Could you check a few things on this drawing? It's one solid part, dimensions in mm from its lowest x, y, z. Round coordinates to 2 decimals unless told otherwise and drop trailing zeros. Loops run counter-clockwise (first coordinate to the right, second up) from the corner with the lowest first, then second, coordinate; pieces in that order, holes last. Notation, with made-up numbers: (-39.5, 68.25) -> (-34.5, 68.25) arc R24 cw to (-34.5, 102.25) -> close; hole circle Ø5 at (15, 62). An arc over 180 degrees is marked (long way). Write each question's results on one line, items separated by ' | '.
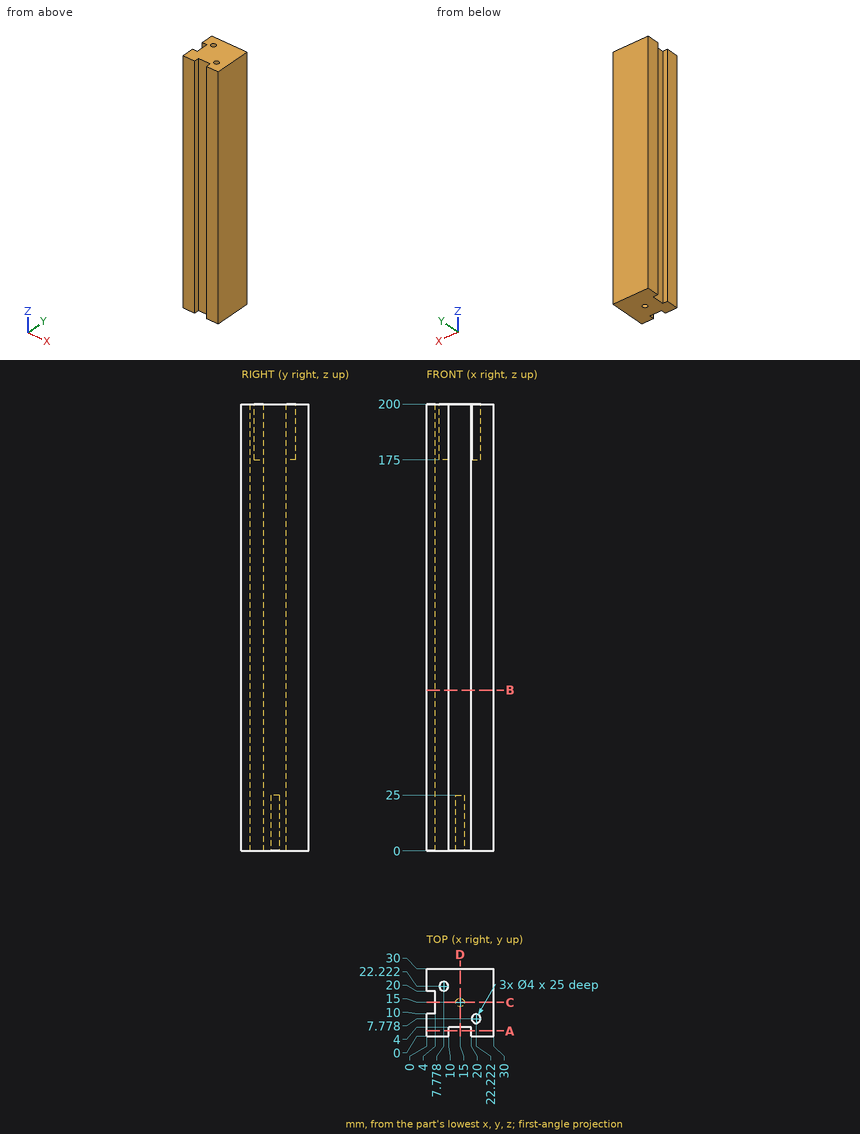
1) I want a section at C-C, the plane y = 15. Write out the boundary of the cut face in (x, z).
Model answer:
outline: (4, 0) -> (13, 0) -> (13, 25) -> (17, 25) -> (17, 0) -> (30, 0) -> (30, 200) -> (4, 200) -> close
2) I'm going to push flat-ended pins straight in: pin 1 (1.5 mm diameter, centred on x = 18.5, z = 34, fed in from -Y); pin 2 (1.2 mm diameter, centred on x = 14.5, y = 15, fed in from -Z); pin 3 (3 mm diameter, centred on x = 7.78, y = 22.22, fed in from +Z). Where does each tip first touch, or does it pass through?
Model answer:
pin 1: stops at y = 4 | pin 2: stops at z = 25 | pin 3: stops at z = 175
3) I want a section at B-B, the plane z = 72. Write out the boundary of the cut face in (x, y).
Model answer:
outline: (0, 0) -> (10, 0) -> (10, 4) -> (20, 4) -> (20, 0) -> (30, 0) -> (30, 30) -> (0, 30) -> (0, 20) -> (4, 20) -> (4, 10) -> (0, 10) -> close
4) I want a section at A-A, the plane y = 2.25. Write out the boundary of the cut face in (x, z).
Model answer:
outline: (0, 0) -> (10, 0) -> (10, 200) -> (0, 200) -> close; (20, 0) -> (30, 0) -> (30, 200) -> (20, 200) -> close
5) I need wall thicknesses on line 1 (Y direction, x = 3, z = 131); line 2 (Y direction, x = 15, z = 5.5); line 3 (X direction, y = 12, z = 23.5). Which ranges of each line are inside material? Lowest first, please.
Model answer:
line 1: y = 0 to 10, 20 to 30 | line 2: y = 4 to 13, 17 to 30 | line 3: x = 4 to 30
